The listing builds one solid part. Answer for the finished solid, in the listing's coordinates (mm). Face numbers are marked on the shaded views. A direction names the side the tool comes from. Round coordinates to 2 decimals unless told otherwise and drop trailing zeros. Loops run counter-clockwise (first coordinate to the right, second up) from the corner with the lowest first, then second, coordinate; pieces in that order, holes last. Notation, with made-up numbers: M 73,89 L 94,89 A25 cw 94,119 Z; hole C 23,47 d3. An arc over 180 degrees is marked long. Put each result on its own line as item: value. Start each with the question number.
(1) Straight lines are drawn through the part: line 1 (Y direction, x = 6.75, z = 1.55); line 2 (Z direction, x = 13.5, y = -16); line 3 (X direction, y = -3, z = 2). For each, find the intervals that lie inside material, in ascending order.
(2) Section A-A, the plane y = -22 is taken. Determine the outline of the cut face in (x, z), then the cut area to 3 significant figures.
(3) Section B-B, the plane x = -3.25 is taken. Determine the outline of the cut face in (y, z), then the cut area to 3 significant figures.
(4) Which of the six approach directions +Z, -Z, +X, -X, +Y, -Y give full straight-line access (tool end or side, diameter ignored) to the marked faces 1, 2, 3 and 4?
(5) Flat-ended cylindrical pins translate along their axes: P1, Ø1.5, axis at x = -2, z = 3.5, coming from the +Y side; P2, Ø2.5, axis at x = -3.5, z = 3, coming from the -Y side; P3, Ø1.5, axis at y = -23.5, z = 3.5, coming from the +X side. Find the tip coordinate at first contact, or state that the pin passes through.
(6) Section C-C, the plane y = 17 is taken. Determine the outline of the cut face in (x, z), then the cut area to 3 significant figures.
```python
from build123d import *

# Parameters (mm, degrees)
F0_W     = 30
F0_H     = 60
F1_DEPTH = 1
F2_W     = 17
F2_H     = 8
F3_DEPTH = 5
F4_R     = 2
F5_DEPTH = 1
F6_R     = 1
F7_R     = 1.6
F8_DEPTH = 3


with BuildPart() as f1:
    # F0 (on Top) → F1 (new body)
    with BuildSketch(Plane.XY):
        Rectangle(F0_W, F0_H)
    extrude(amount=-F1_DEPTH)

    # F2 (on Top) → F3 (join)
    with BuildSketch(Plane.XY):
        Rectangle(F2_W, F2_H)
        with Locations((0, -11)):
            Rectangle(F2_W, F2_H)
        with Locations((0, 11)):
            Rectangle(F2_W, F2_H)
        with Locations((0, -22)):
            Rectangle(F2_W, F2_H)
        with Locations((0, 22)):
            Rectangle(F2_W, F2_H)
    extrude(amount=F3_DEPTH)

    # F4 (on face) → F5 (cut)
    with BuildSketch(Plane.XY.offset(5)):
        Circle(F4_R)
        with Locations((0, 11)):
            Circle(F4_R)
        with Locations((0, 22)):
            Circle(F4_R)
        with Locations((0, -11)):
            Circle(F4_R)
        with Locations((0, -22)):
            Circle(F4_R)
    extrude(amount=-F5_DEPTH, mode=Mode.SUBTRACT)

    # F6
    f6_edges = [f1.edges().sort_by_distance(p)[0] for p in [
        (-8.5, 4, 2.5),
        (8.5, 4, 2.5),
        (8.5, -4, 2.5),
        (-8.5, -4, 2.5),
        (-15, 30, -0.5),
        (15, 30, -0.5),
        (15, -30, -0.5),
        (-15, -30, -0.5),
        (-8.5, -26, 2.5),
        (-8.5, -15, 2.5),
        (-8.5, -7, 2.5),
        (-8.5, 7, 2.5),
        (-8.5, 15, 2.5),
        (-8.5, 18, 2.5),
        (-8.5, 26, 2.5),
        (-8.5, -18, 2.5),
        (8.5, -26, 2.5),
        (8.5, -18, 2.5),
        (8.5, -15, 2.5),
        (8.5, -7, 2.5),
        (8.5, 7, 2.5),
        (8.5, 15, 2.5),
        (8.5, 18, 2.5),
        (8.5, 26, 2.5),
    ]]
    fillet(f6_edges, radius=F6_R)

    # F7 (on face) → F8 (cut)
    with BuildSketch(Plane.XY.offset(4)):
        Circle(F7_R)
        with Locations((0, -11)):
            Circle(F7_R)
        with Locations((0, -22)):
            Circle(F7_R)
        with Locations((0, 11)):
            Circle(F7_R)
        with Locations((0, 22)):
            Circle(F7_R)
    extrude(amount=-F8_DEPTH, mode=Mode.SUBTRACT)


solid = f1.part
```
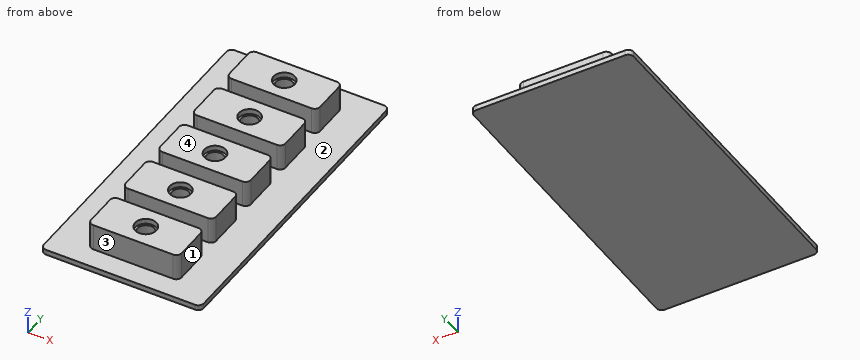
Recorded:
1. line 1: y = -26 to -18, -15 to -7, -4 to 4, 7 to 15, 18 to 26
1. line 2: z = -1 to 0
1. line 3: x = -8.5 to 8.5
2. outline: M -15,-1 L 15,-1 L 15,0 L 8.5,0 L 8.5,5 L 2,5 L 2,4 L 1.6,4 L 1.6,1 L -1.6,1 L -1.6,4 L -2,4 L -2,5 L -8.5,5 L -8.5,0 L -15,0 Z
2. area: 101 mm²
3. outline: M -30,-1 L 30,-1 L 30,0 L 26,0 L 26,5 L 18,5 L 18,0 L 15,0 L 15,5 L 7,5 L 7,0 L 4,0 L 4,5 L -4,5 L -4,0 L -7,0 L -7,5 L -15,5 L -15,0 L -18,0 L -18,5 L -26,5 L -26,0 L -30,0 Z
3. area: 260 mm²
4. face 1: +Z, +X, +Y, -Y
4. face 2: +Z
4. face 3: +Z, +X, -X, -Y
4. face 4: +Z, +X, -X, +Y, -Y
5. P1: stops at y = 26
5. P2: stops at y = -26
5. P3: stops at x = 8.5
6. outline: M -15,-1 L 15,-1 L 15,0 L -15,0 Z
6. area: 30.0 mm²
